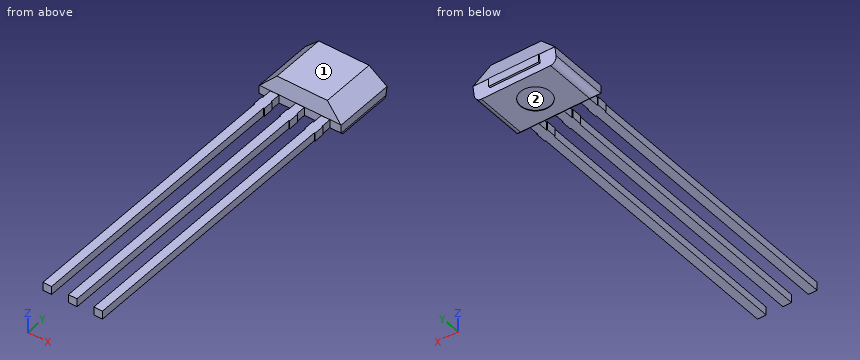
from build123d import *

# Parameters (mm, degrees)
BOSS_EXTRUDE1_DEPTH      = 1.44
BOSS_EXTRUDE1_DEPTH_BACK = 1.58
CUT_EXTRUDE1_START       = -2.045
CUT_EXTRUDE1_DEPTH       = 4.09
SKETCH3_W                = 2.51
SKETCH3_H                = 0.162535045
BOSS_EXTRUDE2_DEPTH      = 0.41
SKETCH4_R                = 0.75
CUT_EXTRUDE2_DEPTH       = 0.025


with BuildPart() as part:
    # Sketch1 → Boss-Extrude1 (new, two sides: drawn at the far end of the back side and taken through both)
    with BuildSketch(Plane(origin=(0, 0, 0), x_dir=(1, 0, 0), z_dir=(0, 1, 0)).offset(-BOSS_EXTRUDE1_DEPTH_BACK)):
        with BuildLine():
            Line((-2.045, 0), (-1.255, -0.79))
            Line((-1.255, -0.79), (1.255, -0.79))
            Line((1.255, -0.79), (2.045, 0))
            Line((2.045, 0), (2.045, 0.41))
            ThreePointArc((2.045, 0.41), (1.95127417, 0.63627417), (1.725, 0.73))
            Line((1.725, 0.73), (-1.725, 0.73))
            ThreePointArc((-1.725, 0.73), (-1.95127417, 0.63627417), (-2.045, 0.41))
            Line((-2.045, 0.41), (-2.045, 0))
        make_face()
    extrude(amount=BOSS_EXTRUDE1_DEPTH + BOSS_EXTRUDE1_DEPTH_BACK)

    # Sketch2 → Cut-Extrude1 (cut)
    with BuildSketch(Plane(origin=(0, 0, 0), x_dir=(0, 0, -1), z_dir=(1, 0, 0)).offset(CUT_EXTRUDE1_START)):
        Polygon((0.41, -1.58), (0.73, -1.58), (0.73, -1.26), align=None)
        Polygon((-0.01, 1.44), (-0.79, 1.44), (-0.79, 1.302464955), align=None)
        Polygon((-0.01, -1.58), (-0.79, -1.442464955), (-0.79, -1.58), align=None)
        Polygon((0.73, 1.311281304), (0.73, 1.44), (0, 1.44), align=None)
    extrude(amount=CUT_EXTRUDE1_DEPTH, mode=Mode.SUBTRACT)

    # Sketch3 → Boss-Extrude2 (add)
    with BuildSketch(Plane.XY):
        Polygon((1.485, -1.58), (1.055, -1.58), (1.055, -2.09), (1.015, -2.09), (1.015, -2.6), (1.055, -2.6), (1.055, -16.53), (1.485, -16.53), (1.485, -2.6), (1.525, -2.6), (1.525, -2.09), (1.485, -2.09), align=None)
        Polygon((0.215, -1.58), (-0.215, -1.58), (-0.215, -2.09), (-0.255, -2.09), (-0.255, -2.6), (-0.215, -2.6), (-0.215, -16.53), (0.215, -16.53), (0.215, -2.6), (0.255, -2.6), (0.255, -2.09), (0.215, -2.09), align=None)
        Polygon((-1.055, -1.58), (-1.485, -1.58), (-1.485, -2.09), (-1.525, -2.09), (-1.525, -2.6), (-1.485, -2.6), (-1.485, -16.53), (-1.055, -16.53), (-1.055, -2.6), (-1.015, -2.6), (-1.015, -2.09), (-1.055, -2.09), align=None)
        with Locations((0, 1.383732478)):
            Rectangle(SKETCH3_W, SKETCH3_H)
    extrude(amount=-BOSS_EXTRUDE2_DEPTH)

    # Sketch4 → Cut-Extrude2 (cut)
    with BuildSketch(Plane(origin=(0, 0, -0.73), x_dir=(-1, 0, 0), z_dir=(0, 0, -1))):
        with Locations((0, 0.025640652)):
            Circle(SKETCH4_R)
    extrude(amount=-CUT_EXTRUDE2_DEPTH, mode=Mode.SUBTRACT)


solid = part.part
The model under review builds one solid part; all positions refer to its coordinate system, in mm. Face numbers are marked on the shaded views. Round coordinates to 2 decimals unless told otherwise and drop trailing zeros. Order: outer loops, then holes, each group sorted by start corner. A loop starts at its lowest first (then second) coordinate and runs counter-clockwise, first axis right, second up. Notation, with made-up numbers: (17, 29) -> (29, 29) arc R21 ccw to (29, 41) -> close; hole circle Ø8 at (50, 37). An arc over 180 degrees is marked (long way). Return JSON: item names as keys, results as strings.
1. Take a section at B-B (x = 0). Write out the cut boundary in (y, z) (3 decimals), then the cut area to 3 significant figures.
Answer block:
{"outline": "(-16.53, -0.41) -> (-1.58, -0.41) -> (-1.26, -0.73) -> (-0.724, -0.73) -> (-0.724, -0.705) -> (0.776, -0.705) -> (0.776, -0.73) -> (1.311, -0.73) -> (1.368, -0.41) -> (1.465, -0.41) -> (1.465, 0) -> (1.44, 0) -> (1.44, 0.01) -> (1.302, 0.79) -> (-1.442, 0.79) -> (-1.58, 0.01) -> (-1.58, 0) -> (-16.53, 0) -> close", "area": "10.5 mm²"}
2. Take a section at D-D (z = 0.6). Write out the cut boundary in (x, y) (3 decimals).
Answer block:
{"outline": "(-1.445, -1.476) -> (1.445, -1.476) -> (1.445, 1.336) -> (-1.445, 1.336) -> close"}
3. For L1, parallel to X at y = -5.5, z = -0.25 (3 decimals); L2, parallel to Z at x = -1.4, y = -6.5; L3, parallel to Y at x = 0.55, z = -0.2 (3 decimals), list the stretches that pass through material, from the lowest coordinate up. Write a range as [from, to].
Answer block:
{"L1": "x = [-1.485, -1.055], [-0.215, 0.215], [1.055, 1.485]", "L2": "z = [-0.41, 0]", "L3": "y = [-1.58, 1.465]"}
4. Insertion check: P1, Ø0.5, axis at y = -2, z = -0.5, coming from the -X side (3 decimals); P2, Ø1.2, axis at x = 0, y = 0, coming from the -Z side (3 decimals); P3, Ø0.5, axis at y = -2.5, z = 0, coming from the +X side (3 decimals). Each pin has a flat end and moves straight along its axis. Give the tip position at first contact, or say it passes through.
Answer block:
{"P1": "stops at x = -1.525", "P2": "stops at z = -0.705", "P3": "stops at x = 1.525"}
5. Take a section at A-A (y = -4.75). Write out the cut boundary in (x, z) (3 decimals), then the cut area to 3 significant figures.
Answer block:
{"outline": "(-1.485, -0.41) -> (-1.055, -0.41) -> (-1.055, 0) -> (-1.485, 0) -> close; (-0.215, -0.41) -> (0.215, -0.41) -> (0.215, 0) -> (-0.215, 0) -> close; (1.055, -0.41) -> (1.485, -0.41) -> (1.485, 0) -> (1.055, 0) -> close", "area": "0.529 mm²"}
6. Take a section at C-C (y = -0.5). Write out the cut boundary in (x, z) (3 decimals).
Answer block:
{"outline": "(-2.045, -0.41) arc R0.32 ccw to (-1.725, -0.73) -> (-0.535, -0.73) -> (-0.535, -0.705) -> (0.535, -0.705) -> (0.535, -0.73) -> (1.725, -0.73) arc R0.32 ccw to (2.045, -0.41) -> (2.045, 0) -> (1.255, 0.79) -> (-1.255, 0.79) -> (-2.045, 0) -> close"}
7. The part is to be moulded in two halves that separate along Y. For the marked faces 1 and 2, say which applies: +Y half, -Y half, draft (parallel to the pull), parting line (faces both ways), or undercut.
Answer block:
{"face 1": "draft", "face 2": "undercut"}
